Input: dimensioned drawing with shaded views. Units: mm. Origin: part minimum x, y, z. A direction names the side the tool comes from. Give positions to 0.01 mm unless a question says otherwise; leave off trailing zeros. Write each loop counter-clockwise with the first axis right and the second up, starting at its lowest first coordinate (ties: lowest second). Pieces come first, ordered by that corner, then holes. Notation, with made-up numbers: (-28, -10) - (8, -10) arc R11 ccw to (8, 4) - close; hole circle Ø10 at (80.25, 43.25). An arc over 180 degrees is marked (long way). Answer as a JSON object with one key per item and string values. Group by question number.
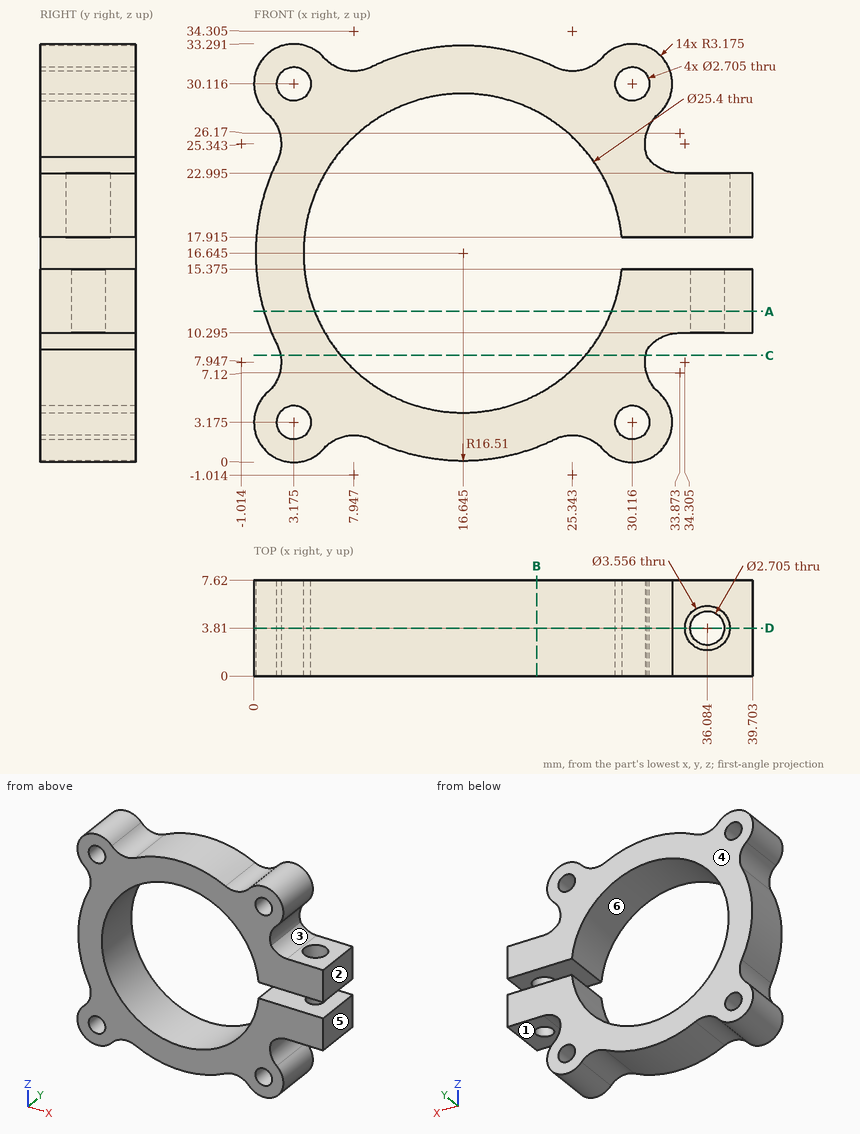
1) Pin query (flat end, axial travel): P1, Ø2.5, axis at x = 3.17, z = 30.12, coming from the +Y side; P2, Ø1.7, axis at x = 36.5, y = 5, coming from the -Z side (1 decimal); P3, Ø4.5, axis at x = 36.08, y = 3.81, coming from the +Z side; P4, Ø4, axis at y = 4.5, z = 7.5, coming from the +X side. Return the tip coordinate at first contact, or that it passes through.
2) Mould query, pull axis X, two halves, no side actions, for the marked faces 4, 5 and 6. Classes: +X half, -X half, draft (parallel to the pull), parting line (faces both ways), or undercut.
3) Line query: line 1 along Z through (x, y) = (37.5, 6.75) (1 decimal); line 2 along X through (y, z) = (1, 3) (1 decimal); line 3 along X through (y, z) = (3.5, 18.5) (1 decimal). Output: solid intervals per line, ascending. Write a range as from..to.
4) Reachability of the marked faces 1, 2 and 3 from +Z, -Z, +X, -X, +Y, -Y: full face, straight path, thin tool, end or side. Return the list, or none.
5) Cut plane B-B on x = 22.5. Return the cut outline in (y, z) (1 decimal).
6) Cut plane A-A on z = 12. Return the cut outline in (x, y) (1 decimal).
7) Cut plane D-D on y = 3.81. Count the separate pieces of the cut face and the enclosed holes in it, and give its area (3 significant figures).
8) Cut plane C-C on z = 8.5. Return the cut outline in (x, y).
Filled in:
{
 "1": {"P1": "passes through", "P2": "stops at z = 10.3", "P3": "stops at z = 23", "P4": "stops at x = 32.28"},
 "2": {"face 4": "draft", "face 5": "+X half", "face 6": "undercut"},
 "3": {"line 1": "z = 10.3..15.4, 17.9..23", "line 2": "x = 0..1.8, 4.5..28.8, 31.5..33.3", "line 3": "x = 0.2..4.1, 29.2..34.3, 37.8..39.7"},
 "4": {"face 1": "-Z, +X, +Y, -Y", "face 2": "+Z, -Z, +X, +Y, -Y", "face 3": "+X, +Y, -Y"},
 "5": {"outline": "(0, 1.2) - (7.6, 1.2) - (7.6, 5.4) - (0, 5.4) - close; (0, 27.9) - (7.6, 27.9) - (7.6, 32.1) - (0, 32.1) - close"},
 "6": {"outline": "(0.8, 0) - (4.8, 0) - (4.8, 7.6) - (0.8, 7.6) - close; (28.5, 0) - (39.7, 0) - (39.7, 7.6) - (28.5, 7.6) - close; hole circle Ø2.7 at (36.1, 3.8)"},
 "7": {"separate pieces": "3", "enclosed holes": "4", "area": "497 mm²"},
 "8": {"outline": "(2.11, 0) - (6.9, 0) - (6.9, 7.62) - (2.11, 7.62) - close; (26.39, 0) - (31.18, 0) - (31.18, 7.62) - (26.39, 7.62) - close"}
}
